from build123d import *

# Parameters (mm, degrees)
F0_R     = 2
F1_DEPTH = 8
F2_DEPTH = 2
F3_R     = 20
F4_R     = 1
F6_D     = 4
F7_R     = 3.99999


# Not quite as in the source:
# - a fillet or chamfer is up to 0.001 mm smaller than in the source, because OpenCascade refuses the exact size
# - a feature names something its author has since deleted; it is built from what else it names


with BuildPart() as f1:
    # F0 (on Front) → F1 (new body)
    with BuildSketch(Plane.XZ):
        with BuildLine():
            Line((15.1970139668, 6.8636525628), (6.0880650012, 27.0320429916))
            ThreePointArc((6.0880650012, 27.0320429916), (0, 30.9626), (-6.0880650012, 27.0320429916))
            Line((-6.0880650012, 27.0320429916), (-15.1970139668, 6.8636525628))
            ThreePointArc((-15.1970139668, 6.8636525628), (-16.6751, 0), (-15.1970139668, -6.8636525628))
            Line((-15.1970139668, -6.8636525628), (-11.75, -14.4957870449))
            Line((-11.75, -14.4957870449), (-9.75, -18.9240455641))
            Line((-9.75, -18.9240455641), (-6.1194285683, -26.9626))
            Line((-6.1194285683, -26.9626), (6.1194285683, -26.9626))
            Line((6.1194285683, -26.9626), (9.75, -18.9240455641))
            Line((9.75, -18.9240455641), (11.75, -14.4957870449))
            Line((11.75, -14.4957870449), (15.1970139668, -6.8636525628))
            ThreePointArc((15.1970139668, -6.8636525628), (16.6751, 0), (15.1970139668, 6.8636525628))
        make_face()
        with Locations((0, -24.2824)):
            Circle(F0_R, mode=Mode.SUBTRACT)
        with BuildLine():
            Line((-13.3742945868, 6.0404308054), (-6.0462846285, 22.2655920687))
            ThreePointArc((-6.0462846285, 22.2655920687), (-5.1436901116, 22.8539427752), (-4.2309206889, 22.2815046593))
            ThreePointArc((-4.2309206889, 22.2815046593), (0, 19.6022), (4.2309206889, 22.2815046593))
            ThreePointArc((4.2309206889, 22.2815046593), (5.1436901116, 22.8539427752), (6.0462846285, 22.2655920687))
            Line((6.0462846285, 22.2655920687), (13.3742945868, 6.0404308054))
            ThreePointArc((13.3742945868, 6.0404308054), (14.6751, 0), (13.3742945868, -6.0404308054))
            Line((13.3742945868, -6.0404308054), (6.0462846285, -22.2655920687))
            ThreePointArc((6.0462846285, -22.2655920687), (5.1436901116, -22.8539427752), (4.2309206889, -22.2815046593))
            ThreePointArc((4.2309206889, -22.2815046593), (0, -19.6022), (-4.2309206889, -22.2815046593))
            ThreePointArc((-4.2309206889, -22.2815046593), (-5.1436901116, -22.8539427752), (-6.0462846285, -22.2655920687))
            Line((-6.0462846285, -22.2655920687), (-13.3742945868, -6.0404308054))
            ThreePointArc((-13.3742945868, -6.0404308054), (-14.6751, 0), (-13.3742945868, 6.0404308054))
        make_face(mode=Mode.SUBTRACT)
        with Locations((0, 24.2824)):
            Circle(F0_R, mode=Mode.SUBTRACT)
        Polygon((11.75, -34.9626), (11.75, -14.4957870449), (9.75, -18.9240455641), (9.75, -26.9626), (6.1194285683, -26.9626), (-6.1194285683, -26.9626), (-9.75, -26.9626), (-9.75, -18.9240455641), (-11.75, -14.4957870449), (-11.75, -34.9626), align=None)
    extrude(amount=F1_DEPTH)

    # F0 (on Front) → F2 (join)
    with BuildSketch(Plane.XZ):
        with BuildLine():
            ThreePointArc((-4.2309206889, 22.2815046593), (-5.1436901116, 22.8539427752), (-6.0462846285, 22.2655920687))
            Line((-6.0462846285, 22.2655920687), (-13.3742945868, 6.0404308054))
            ThreePointArc((-13.3742945868, 6.0404308054), (-14.6751, 0), (-13.3742945868, -6.0404308054))
            Line((-13.3742945868, -6.0404308054), (-6.0462846285, -22.2655920687))
            ThreePointArc((-6.0462846285, -22.2655920687), (-5.1436901116, -22.8539427752), (-4.2309206889, -22.2815046593))
            ThreePointArc((-4.2309206889, -22.2815046593), (0, -19.6022), (4.2309206889, -22.2815046593))
            ThreePointArc((4.2309206889, -22.2815046593), (5.1436901116, -22.8539427752), (6.0462846285, -22.2655920687))
            Line((6.0462846285, -22.2655920687), (13.3742945868, -6.0404308054))
            ThreePointArc((13.3742945868, -6.0404308054), (14.6751, 0), (13.3742945868, 6.0404308054))
            Line((13.3742945868, 6.0404308054), (6.0462846285, 22.2655920687))
            ThreePointArc((6.0462846285, 22.2655920687), (5.1436901116, 22.8539427752), (4.2309206889, 22.2815046593))
            ThreePointArc((4.2309206889, 22.2815046593), (0, 19.6022), (-4.2309206889, 22.2815046593))
        make_face()
        Polygon((11.75, -34.9626), (11.75, -14.4957870449), (9.75, -18.9240455641), (9.75, -26.9626), (6.1194285683, -26.9626), (-6.1194285683, -26.9626), (-9.75, -26.9626), (-9.75, -18.9240455641), (-11.75, -14.4957870449), (-11.75, -34.9626), align=None)
        Polygon((-6.1194285683, -26.9626), (-9.75, -18.9240455641), (-9.75, -26.9626), align=None)
        Polygon((9.75, -26.9626), (9.75, -18.9240455641), (6.1194285683, -26.9626), align=None)
    extrude(amount=F2_DEPTH)

    # F3
    f3_edges = [f1.edges().sort_by_distance(p)[0] for p in [
        (11.75, -4, -14.495787),
        (-11.75, -4, -14.495787),
    ]]
    fillet(f3_edges, radius=F3_R)

    # F4
    f4_edges = [f1.edges().sort_by_distance(p)[0] for p in [
        (9.75, -5, -18.924046),
        (-9.75, -5, -18.924046),
    ]]
    fillet(f4_edges, radius=F4_R)

    # F6 (through all)
    with Locations(Plane.YZ.offset(11.75)):
        with Locations((-4, -30.9626)):
            Hole(F6_D / 2)

    # F7 (radius 4 in the source; OpenCascade refuses exactly that, so slightly less here)
    f7_edges = [f1.edges().sort_by_distance(p)[0] for p in [
        (0, -8, -34.9626),
        (7.934714, -8, -26.9626),
        (-7.934714, -8, -26.9626),
    ]]
    fillet(f7_edges, radius=F7_R)


solid = f1.part
Verification items for the finished model (mm, model axes). A direction names the side the tool comes from. Round coordinates to 2 decimals unless told otherwise and drop trailing zeros. Loops run counter-clockwise (first coordinate to the right, second up) from the corner with the lowest first, then second, coordinate; pieces in that order, holes last. Notation, with made-up numbers: (55.25, 0) - (101.25, 0) arc R9 cw to (101.25, 5) - close; hole circle Ø2 at (-7.75, -32.5). An arc over 180 degrees is marked (long way). Use one line per item in the form item = value.
1. Section check B-B on z = 14.5. Record the cut outline in (x, y), and give its area (3 significant figures).
A:
outline = (-11.75, -8) - (-9.55, -8) - (-9.55, -2) - (9.55, -2) - (9.55, -8) - (11.75, -8) - (11.75, 0) - (-11.75, 0) - close
area = 73.3 mm²
2. Section check D-D on y = -2.75. Give the number of separate pieces and of enclosed holes in the cut face, and give its area (3 significant figures).
A:
separate_pieces = 2
enclosed_holes = 5
area = 531 mm²
3. Gauge pin test, flat ends, axial feed: pin 1 Ø1.8 at (x, z) = (-7.5, -24) entering from -Y; pin 2 Ø2 at (x, y) = (-8.5, -3) entering from +Z; pin 3 Ø1 at (x, y) = (7.5, -3.5) entering from +Z; pin 4 Ø1 at (x, y) = (-13, -6) entering from +Z. Record the tip position at first contact, or that the pin passes through.
A:
pin_1 = -8
pin_2 = 23.91
pin_3 = 25.01
pin_4 = 12.84
4. Section check A-A on x = 0. Record the cut outline in (y, z), and give its area (3 significant figures).
A:
outline = (-8, -30.96) arc R4 ccw to (-4, -34.96) - (0, -34.96) - (0, -26.28) - (-8, -26.28) - close; (-8, -22.28) - (0, -22.28) - (0, 22.28) - (-8, 22.28) - (-8, 19.6) - (-2, 19.6) - (-2, -19.6) - (-8, -19.6) - close; (-8, 26.28) - (0, 26.28) - (0, 30.96) - (-8, 30.96) - close; hole circle Ø4 at (-4, -30.96)
area = 212 mm²
5. Scan lines: probe 1 along Z at (x, y) = (0, -1.75); probe 2 along Z at (x, y) = (0, -4.75); probe 3 along Z at (x, y) = (0, -5). Record each from-to range of solid material in increasing order.
A:
probe_1 = -34.96 to -26.28, -22.28 to 22.28, 26.28 to 30.96
probe_2 = -34.89 to -32.82, -29.11 to -26.28, -22.28 to -19.6, 19.6 to 22.28, 26.28 to 30.96
probe_3 = -34.84 to -32.69, -29.23 to -26.28, -22.28 to -19.6, 19.6 to 22.28, 26.28 to 30.96
6. Access from +Z, -Z, +X, -X, +Y, -Y to the whole of each face (thin tool, end or side, straight path). Record for faces 1 (the flat face through (-8, -3, -26.963)), 2 (the flat face through (-11.75, -4, -27)), 3 (the flat face through (10.706, -3.944, 16.807)).
A:
face_1 = -Y
face_2 = -Z, -X, +Y, -Y
face_3 = +Z, +X, +Y, -Y
7. Draft check along Z on faces 4 (the cylindrical face through (0.16, -6.86, -33.76)), 5 (the cylindrical face through (0.11, -3.94, 30.96)), 6 (the flat face through (8, -2, -25)), 7 (the cylindrical face through (16.675, -3.944, -0.099)). Enter one of: pulls with the +Z half, pulls with the -Z half, needs draft (parallel to the pull), parting line crosses it, or undercut.
A:
face_4 = pulls with the -Z half
face_5 = pulls with the +Z half
face_6 = undercut
face_7 = parting line crosses it
